```python
from build123d import *

# Parameters (mm, degrees)
F0_R      = 20
F1_DEPTH  = 32
F2_R      = 18.5
F3_DEPTH  = 2
F4_R      = 19
F5_DEPTH  = 11
F6_R      = 14
F7_DEPTH  = 2
F8_R      = 14.7
F9_DEPTH  = 1.35
F10_R     = 14
F11_DEPTH = 21.5
F12_R     = 11
F13_DEPTH = 18
F14_R     = 7
F15_DEPTH = 25
F17_D     = 4.4
F17_DEPTH = 15
F17_TIP   = 1.3218933619
F19_START = -10
F18_W     = 20
F18_H     = 43.6686427468
F19_DEPTH = 8
F20_SIZE  = 0.5


with BuildPart() as f1:
    # F0 (on Top) → F1 (new body)
    with BuildSketch(Plane.XY):
        Circle(F0_R)
    extrude(amount=F1_DEPTH)

    # F2 (on face) → F3 (join)
    with BuildSketch(Plane.XY.offset(32)):
        Circle(F2_R)
    extrude(amount=F3_DEPTH)

    # F4 (on face) → F5 (join)
    with BuildSketch(Plane.XY.offset(34)):
        Circle(F4_R)
    extrude(amount=F5_DEPTH)

    # F6 (on face) → F7 (cut)
    with BuildSketch(Plane.XY.offset(45)):
        Circle(F6_R)
    extrude(amount=-F7_DEPTH, mode=Mode.SUBTRACT)

    # F8 (on face) → F9 (cut)
    with BuildSketch(Plane.XY.offset(43)):
        Circle(F8_R)
    extrude(amount=-F9_DEPTH, mode=Mode.SUBTRACT)

    # F10 (on face) → F11 (cut)
    with BuildSketch(Plane.XY.offset(41.65)):
        Circle(F10_R)
    extrude(amount=-F11_DEPTH, mode=Mode.SUBTRACT)

    # F12 (on face) → F13 (cut)
    with BuildSketch(Plane.XY.offset(20.15)):
        Circle(F12_R)
    extrude(amount=-F13_DEPTH, mode=Mode.SUBTRACT)

    # F14 (on face) → F15 (cut)
    with BuildSketch(Plane.XY.offset(2.15)):
        Circle(F14_R)
    extrude(amount=-F15_DEPTH, mode=Mode.SUBTRACT)

    # F17
    with Locations(Plane(origin=(0, 0, 0), x_dir=(1, 0, 0), z_dir=(0, 0, -1))):
        with Locations((-16, 0), (0, 16), (16, 0), (0, -16)):
            Hole(F17_D / 2, depth=F17_DEPTH)
            with Locations((0, 0, -(F17_DEPTH + F17_TIP / 2))):  # 118° drill point
                Cone(0, F17_D / 2, F17_TIP, mode=Mode.SUBTRACT)

    # F18 (on face) → F19 (cut)
    with BuildSketch(Plane(origin=(0, 0, 0), x_dir=(1, 0, 0), z_dir=(0, 0, -1)).offset(F19_START)):
        with Locations((18, -0.2762433141)):
            Rectangle(F18_W, F18_H)
    extrude(amount=-F19_DEPTH, mode=Mode.SUBTRACT)

    # F20
    f20_edges = [f1.edges().sort_by_distance(p)[0] for p in [
        (-20, 0, 0),
        (-19, 0, 45),
    ]]
    chamfer(f20_edges, length=F20_SIZE)


solid = f1.part
```
Design review of the part built by this model. Coordinates are the model's own, in mm. A direction names the side the tool comes from. Give positions to 0.01 mm unless a question says otherwise; leave off trailing zeros. Order: outer loops, then holes, each group sorted by start corner. A loop starts at its lowest first (then second) coordinate and runs counter-clockwise, first axis right, second up. Notation, with made-up numbers: (72, -16) -> (102, -16) arc R17 cw to (102, -2) -> close; hole circle Ø5 at (21, 12.5). An arc over 180 degrees is marked (long way). Write item = value, one per line. Start each with the question number.
(1) We need section C-C on x = 15.5. State how many separate pieces and enclosed holes the cut face has, plus the area to 3 significant figures.
(2) We need section A-A on z = 12. Write out the cut boundary in (x, y).
(3) To check wall thickness, follow line 1 along Y through (x, z) = (0, 0.95); line 2 along Y through (x, z) = (0, 11.5); line 3 along Z through (x, y) = (11, 5). State the ranges of each line that lie inside material, in increasing order.
(4) Mouldability with a two-part tool opening along Z and no side actions: class faces 4 (the face through (8, 0, 0)), 5 (the face through (12, -8, 41.65)), 6 (the face through (6.2, -9.3, 20.15)), 7 (the face through (0.477, -13.852, 7.605)) as +Z half, -Z half, draft (parallel to the pull), parting line (faces both ways), or undercut.
(5) For pin 1 (12 mm diameter, centred on x = 10, z = 23, fed in from -Y); pin 2 (12 mm diameter, centred on x = -2.5, y = 3.5, fed in from +Z); pin 3 (2.5 mm diameter, centred on y = -13, z = 12, fed in from +X); pin 4 (6 mm diameter, centred on x = -6.5, y = 9, fed in from +Z), all flat-tipped, find the tip position at first contact; note any pin that passes through.
(6) For faces 1 (the face through (-18.032, 0.843, 7.605)), 2 (the face through (7.2, 0.2, 2.15)), 3 (the face through (8, 13, 14)), list the 3-axis set-ups (+Z, -Z, +X, -X, +Y, -Y) from which the entire face can be reached by the end or side of a thin tool; tool diameter is ignored.
(7) We need section B-B on z = 36.5. Write out the cut boundary in (x, y).
Numbers:
q1.separate_pieces = 3
q1.enclosed_holes = 0
q1.area = 845 mm^2
q2.outline = (8, -18.33) -> (8, -7.55) arc R11 cw (long way) to (8, 7.55) -> (8, 18.33) arc R20 ccw (long way) to start; hole circle Ø4.4 at (-16, 0); hole circle Ø4.4 at (0, -16); hole circle Ø4.4 at (0, 16)
q3.line_1 = -20 to -18.2, -13.8 to -7, 7 to 13.8, 18.2 to 20
q3.line_2 = -20 to -18.2, -13.8 to -11, 11 to 13.8, 18.2 to 20
q3.line_3 = 0 to 10, 18 to 20.15
q4.face_4 = -Z half
q4.face_5 = undercut
q4.face_6 = +Z half
q4.face_7 = draft
q5.pin_1 = -19.6
q5.pin_2 = 2.15
q5.pin_3 = 8
q5.pin_4 = 45
q6.face_1 = -Z
q6.face_2 = +Z
q6.face_3 = +X, +Y, -Y
q7.outline = circle Ø38 at (0, 0); hole circle Ø28 at (0, 0)
